Read the model definition and answer for the solid it produces. Units are mm, in the model's axes. Face numbers are marked on the shaded views. Give positions to 0.01 mm unless a question says otherwise; leave off trailing zeros. Write each loop counter-clockwise with the first axis right and the second up, starting at its lowest first coordinate (ties: lowest second). Pieces come first, ordered by that corner, then holes. Notation, with made-up numbers: (18, 82) -> (37, 82) arc R16 ccw to (37, 108) -> close; hole circle Ø9 at (-18, 68.5). An arc over 180 degrees is marked (long way). Use a Markdown table: item, result.
from build123d import *

# Parameters (mm, degrees)
F0_R     = 12.5
F1_DEPTH = 3.3
F2_DEPTH = 1.5
F3_DEPTH = 1
F4_D     = 3.5
F5_D     = 2.6


with BuildPart() as f1:
    # F0 (on Top) → F1 (new body)
    with BuildSketch(Plane.XY):
        with BuildLine():
            Line((-13.75, -20), (13.75, -20))
            Line((13.75, -20), (13.75, -17))
            ThreePointArc((13.75, -17), (14.701903, -14.701903), (17, -13.75))
            Line((17, -13.75), (20, -13.75))
            Line((20, -13.75), (20, 13.75))
            Line((20, 13.75), (17, 13.75))
            ThreePointArc((17, 13.75), (14.701903, 14.701903), (13.75, 17))
            Line((13.75, 17), (13.75, 20))
            Line((13.75, 20), (-13.75, 20))
            Line((-13.75, 20), (-13.75, 17))
            ThreePointArc((-13.75, 17), (-14.701903, 14.701903), (-17, 13.75))
            Line((-17, 13.75), (-20, 13.75))
            Line((-20, 13.75), (-20, -13.75))
            Line((-20, -13.75), (-17, -13.75))
            ThreePointArc((-17, -13.75), (-14.701903, -14.701903), (-13.75, -17))
            Line((-13.75, -17), (-13.75, -20))
        make_face()
        Circle(F0_R, mode=Mode.SUBTRACT)
    extrude(amount=F1_DEPTH)

    # F0 (on Top) → F2 (join)
    with BuildSketch(Plane.XY):
        Circle(F0_R)
    extrude(amount=F2_DEPTH)

    # F0 (on Top) → F3 (join)
    with BuildSketch(Plane.XY):
        with BuildLine():
            Line((20, -13.75), (20, -20))
            ThreePointArc((20, -20), (28.271859, 0), (20, 20))
            Line((20, 20), (20, 13.75))
            Line((20, 13.75), (20, -13.75))
        make_face()
        with BuildLine():
            Line((20, 13.75), (20, 20))
            Line((20, 20), (13.75, 20))
            Line((13.75, 20), (13.75, 17))
            ThreePointArc((13.75, 17), (14.701903, 14.701903), (17, 13.75))
            Line((17, 13.75), (20, 13.75))
        make_face()
        with BuildLine():
            Line((13.75, -20), (20, -20))
            Line((20, -20), (20, -13.75))
            Line((20, -13.75), (17, -13.75))
            ThreePointArc((17, -13.75), (14.701903, -14.701903), (13.75, -17))
            Line((13.75, -17), (13.75, -20))
        make_face()
        with BuildLine():
            Line((-13.75, 17), (-13.75, 20))
            Line((-13.75, 20), (-20, 20))
            Line((-20, 20), (-20, 13.75))
            Line((-20, 13.75), (-17, 13.75))
            ThreePointArc((-17, 13.75), (-14.701903, 14.701903), (-13.75, 17))
        make_face()
        with BuildLine():
            ThreePointArc((-20, 20), (-28.273493, 0), (-20, -20))
            Line((-20, -20), (-20, -13.75))
            Line((-20, -13.75), (-20, 13.75))
            Line((-20, 13.75), (-20, 20))
        make_face()
        with BuildLine():
            Line((-20, -20), (-13.75, -20))
            Line((-13.75, -20), (-13.75, -17))
            ThreePointArc((-13.75, -17), (-14.701903, -14.701903), (-17, -13.75))
            Line((-17, -13.75), (-20, -13.75))
            Line((-20, -13.75), (-20, -20))
        make_face()
    extrude(amount=F3_DEPTH)

    # F4 (through all)
    with Locations(Plane(origin=(0, 0, 0), x_dir=(1, 0, 0), z_dir=(0, 0, -1))):
        with Locations((17, 17), (-17, 17), (-17, -17), (17, -17)):
            Hole(F4_D / 2)

    # F5 (through all)
    with Locations(Plane(origin=(0, 0, 0), x_dir=(1, 0, 0), z_dir=(0, 0, -1))):
        with Locations((-3.063159, 16.5), (3.136841, 16.5), (3.136841, -16.5), (-3.063159, -16.5)):
            Hole(F5_D / 2)


solid = f1.part
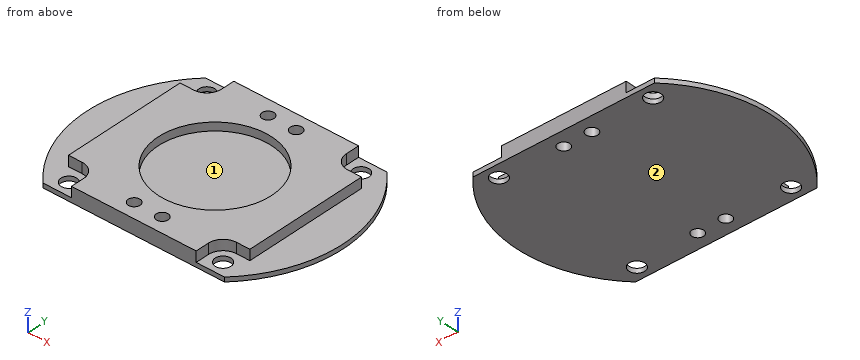
Item 1: Straight lines are drawn through the part: line 1 along Y through (x, z) = (-17, 0.55); line 2 along Y through (x, z) = (3, 1.25); line 3 along X through (y, z) = (-18, 0.7). For each, find the intervals that lie inside material, in ascending order. Write a range as [from, to].
Return value:
| item | result |
|---|---|
| line 1 | [-20, -18.75], [-15.25, 15.25], [18.75, 20] |
| line 2 | [-20, -17.79], [-15.21, 15.21], [17.79, 20] |
| line 3 | [-21.81, -18.44], [-15.56, 15.56], [18.44, 21.81] |
Item 2: A cutting plane is placed at B-B (y = 0). Give the vertices of the cut face in (x, z), then the cut area to 3 significant figures.
Return value:
| item | result |
|---|---|
| outline | (-28.27, 0) -> (28.27, 0) -> (28.27, 1) -> (20, 1) -> (20, 3.3) -> (12.5, 3.3) -> (12.5, 1.5) -> (-12.5, 1.5) -> (-12.5, 3.3) -> (-20, 3.3) -> (-20, 1) -> (-28.27, 1) -> close |
| area | 104 mm^2 |
Item 3: A cutting plane is placed at A-A (z = 2.3). Give the vertices of the cut face in (x, y), then the cut area to 3 significant figures.
Return value:
| item | result |
|---|---|
| outline | (-20, -13.75) -> (-17, -13.75) arc R3.25 cw to (-13.75, -17) -> (-13.75, -20) -> (13.75, -20) -> (13.75, -17) arc R3.25 cw to (17, -13.75) -> (20, -13.75) -> (20, 13.75) -> (17, 13.75) arc R3.25 cw to (13.75, 17) -> (13.75, 20) -> (-13.75, 20) -> (-13.75, 17) arc R3.25 cw to (-17, 13.75) -> (-20, 13.75) -> close; hole circle Ø25 at (0, 0); hole circle Ø2.6 at (-3.06, -16.5); hole circle Ø2.6 at (-3.06, 16.5); hole circle Ø2.6 at (3.14, -16.5); hole circle Ø2.6 at (3.14, 16.5) |
| area | 941 mm^2 |
Item 4: Each of these flat-tipped pins is pushed along its axis until it touches: P1, Ø6, axis at x = 5, y = -5.5, coming from the +Z side; P2, Ø1.8, axis at y = -5.5, z = 2.5, coming from the -X side; P3, Ø1.8, axis at y = 19, z = 1.5, coming from the +X side. Where does it stop, or does it pass through?
Return value:
| item | result |
|---|---|
| P1 | z = 1.5 |
| P2 | x = -20 |
| P3 | x = 21.6 |
Item 5: A cutting plane is placed at C-C (x = -7.5). Give the vertices of the cut face in (y, z), then the cut area to 3 significant figures.
Return value:
| item | result |
|---|---|
| outline | (-20, 0) -> (20, 0) -> (20, 3.3) -> (10, 3.3) -> (10, 1.5) -> (-10, 1.5) -> (-10, 3.3) -> (-20, 3.3) -> close |
| area | 96.0 mm^2 |
Item 6: For a pull along Y with two mould halves and no side action, classify the marked faces 1 and 2 as +Y half, -Y half, draft (parallel to the pull), parting line (faces both ways), or undercut.
Return value:
| item | result |
|---|---|
| face 1 | undercut |
| face 2 | draft |
Item 7: A cutting plane is placed at D-D (x = 0). Give the vertices of the cut face in (y, z).
Return value:
| item | result |
|---|---|
| outline | (-20, 0) -> (20, 0) -> (20, 3.3) -> (12.5, 3.3) -> (12.5, 1.5) -> (-12.5, 1.5) -> (-12.5, 3.3) -> (-20, 3.3) -> close |
